Part model, mm, in its own coordinate system. Face numbers are marked on the shaded views. A direction names the side the tool comes from. Give positions to 0.01 mm unless a question says otherwise; leave off trailing zeros. Write each loop counter-clockwise with the first axis right and the second up, starting at its lowest first coordinate (ties: lowest second). Pieces come first, ordered by that corner, then holes. Notation, with made-up numbers: M 17.25,21.25 L 51.25,21.25 A6 ccw 51.25,27.25 Z; hole C -35.5,-31.5 d10. An arc over 180 degrees is marked long. Write item = value, one per line. Start each with the question number.
from build123d import *

# Parameters (mm, degrees)
F0_W     = 50.8
F0_H     = 63.5
F0_R     = 6.35
F1_DEPTH = 25.4
F2_R     = 0.79375
F3_DEPTH = 50.801
F4_R     = 2.413
F5_DEPTH = 25.4


with BuildPart() as f1:
    # F0 (on Front) → F1 (new body)
    with BuildSketch(Plane.XZ):
        with Locations((0, 12.7)):
            Rectangle(F0_W, F0_H)
        with Locations((-16.51, -10.16)):
            Circle(F0_R, mode=Mode.SUBTRACT)
        Polygon((0, -9.165436), (-7.9375, -4.582718), (-7.9375, 4.582718), (0, 9.165436), (7.9375, 4.582718), (7.9375, -4.582718), align=None, mode=Mode.SUBTRACT)
        with Locations((16.51, -10.16)):
            Circle(F0_R, mode=Mode.SUBTRACT)
    extrude(amount=-F1_DEPTH)

    # F2 (on face) → F3 (cut, through all)
    with BuildSketch(Plane.YZ.offset(25.4)):
        with Locations((12.7, -11.43)):
            Circle(F2_R)
        with Locations((12.7, 0)):
            Circle(F2_R)
    extrude(amount=-F3_DEPTH, mode=Mode.SUBTRACT)

    # F4 (on face) → F5 (cut)
    with BuildSketch(Plane.XY.offset(44.45)):
        with Locations((12.7, 12.7)):
            Circle(F4_R)
        with Locations((-12.7, 12.7)):
            Circle(F4_R)
    extrude(amount=-F5_DEPTH, mode=Mode.SUBTRACT)


solid = f1.part
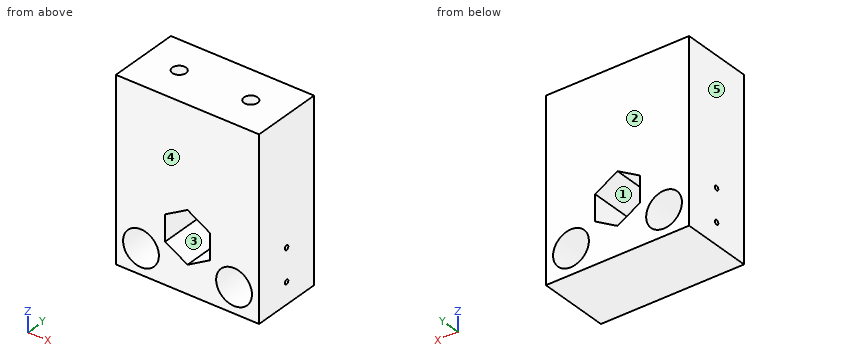
Q1. Two-plate mould, pull along X, no slides. Class the marked faces 3, 4 and 5: +X half, -X half, draft (parallel to the pull), parting line (faces both ways), or undercut.
Q2. Slice it at A-A (x = -12.7). Give the cut face in (y, z), and give its area (3 significant figures).
Q3. Slice it at B-B (z = 1.5). Give the cut face in (x, y).
Q4. Drop a flat-ended pin along its axis: P1, Ø4, axis at x = 12.7, y = 12.7, coming from the +Z side. Give the stop position or say it passes through.
Q5. Slice it at C-C (y = 7.5). Give the cut face in (x, z).
Q6. Slice it at D-D (z = 38). Give the cut face in (x, y).
Q7. Probe line 1 along Y through (x, z) = (-24.45, -11.43); line 2 along X through (y, z) = (16.75, 4.5); line 3 along Y through (x, z) = (-12.7, 38.75). List the from-to ranges inside material, lowest first.
Q8. Tool access for the marked faces 1 and 2: list every direction of +Z, -Z, +X, -X, +Y, -Y with a clear straight run to the whole face (end or side of a thin tool).
Working result:
q1.face_3 = undercut
q1.face_4 = draft
q1.face_5 = -X half
q2.outline = M 0,-19.05 L 25.4,-19.05 L 25.4,-15.24 L 0,-15.24 Z; M 0,-5.08 L 25.4,-5.08 L 25.4,44.45 L 15.11,44.45 L 15.11,19.05 L 10.29,19.05 L 10.29,44.45 L 0,44.45 Z; hole C 12.7,0 d1.59
q2.area = 1,230 mm2
q3.outline = M -25.4,0 L -7.94,0 L -7.94,25.4 L -25.4,25.4 Z; M 7.94,0 L 25.4,0 L 25.4,25.4 L 7.94,25.4 Z
q4.P1 = 19.05
q5.outline = M -25.4,-19.05 L 25.4,-19.05 L 25.4,44.45 L -25.4,44.45 Z; hole C -16.51,-10.16 d12.7; hole M -7.94,-4.58 L 0,-9.17 L 7.94,-4.58 L 7.94,4.58 L 0,9.17 L -7.94,4.58 Z; hole C 16.51,-10.16 d12.7
q6.outline = M -25.4,0 L 25.4,0 L 25.4,25.4 L -25.4,25.4 Z; hole C -12.7,12.7 d4.83; hole C 12.7,12.7 d4.83
q7.line_1 = 0 to 11.91, 13.49 to 25.4
q7.line_2 = -25.4 to -7.94, 7.94 to 25.4
q7.line_3 = 0 to 10.29, 15.11 to 25.4
q8.face_1 = +Y, -Y
q8.face_2 = +Z, -Z, +X, -X, +Y
